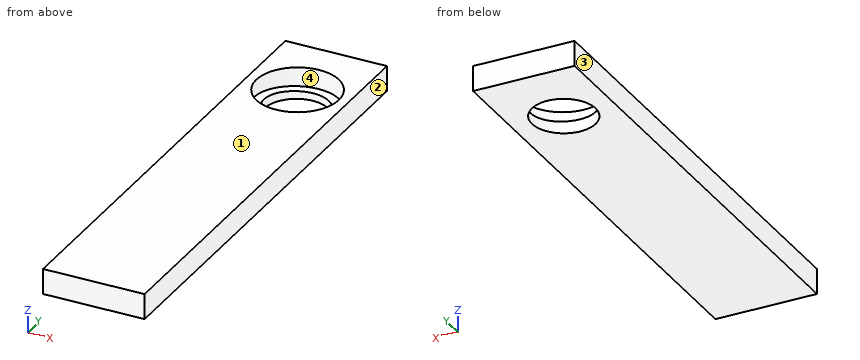
from build123d import *

# Parameters (mm, degrees)
SKETCH1_W           = 80
SKETCH1_H           = 372
BOSS_EXTRUDE1_DEPTH = 20
SKETCH4_R           = 32.5
CUT_EXTRUDE2_DEPTH  = 193.049397179
SKETCH5_R           = 25
CUT_EXTRUDE3_DEPTH  = 193.049397179


with BuildPart() as part:
    # Sketch1 → Boss-Extrude1 (new body)
    with BuildSketch(Plane.XY):
        Rectangle(SKETCH1_W, SKETCH1_H)
    extrude(amount=BOSS_EXTRUDE1_DEPTH)

    # Sketch4 → Cut-Extrude2 (cut, through all)
    with BuildSketch(Plane(origin=(0, 1.135010798, 16.231410618), x_dir=(1, 0, 0), z_dir=(0, -0.06975647374412888, -0.997564050259824))):
        with Locations(Location((0, -124.995505595, 0), (0, 0, 270))):
            Circle(SKETCH4_R)
    extrude(amount=-CUT_EXTRUDE2_DEPTH, mode=Mode.SUBTRACT)

    # Sketch5 → Cut-Extrude3 (cut, through all)
    with BuildSketch(Plane(origin=(0, 1.135010798, 16.231410618), x_dir=(1, 0, 0), z_dir=(0, 0.06975647374412888, 0.9975640502598241))):
        with Locations(Location((0, 124.297940858, 0), (0, 0, 270))):
            Circle(SKETCH5_R)
    extrude(amount=-CUT_EXTRUDE3_DEPTH, mode=Mode.SUBTRACT)


solid = part.part
The model under review builds one solid part; all positions refer to its coordinate system, in mm. Face numbers are marked on the shaded views. Round coordinates to 2 decimals unless told otherwise and drop trailing zeros. Write each loop counter-clockwise with the first axis right and the second up, starting at its lowest first coordinate (ties: lowest second). Pieces come first, ordered by that corner, then holes. Notation, with made-up numbers: (44, -30.5) - (68, -30.5) arc R11 ccw to (68, -12.5) - close; hole circle Ø11 at (35.25, 57.5). An arc over 180 degrees is marked (long way). One line per item, written item: value. Start each with the question number.
1. Consider section B-B on x = -17.5. Write out the cut boundary in (y, z), and give its area (3 significant figures).
2. To check wall thickness, follow L1, parallel to Y at x = 20, z = 11.75; L2, parallel to Y at x = 6, z = 2.5; L3, parallel to X at y = 98, z = 11.75. State the ranges of each line that lie inside material, in increasing order. Write a range as from..to.
3. Consider section A-A on x = 18. Write out the cut boundary in (y, z), and give its area (3 significant figures).
4. The part is to be moulded in two halves that separate along X. For the marked faces 1, 2, 3 and 4, say which applies: released by +X, released by -X, zero draft, split by the parting line, or undercut.
Checks:
1. outline: (-186, 0) - (106.7, 0) - (107.32, 8.81) - (98.51, 9.42) - (99.25, 20) - (-186, 20) - close; (142.5, 0) - (186, 0) - (186, 20) - (154.15, 20) - (153.15, 5.6) - (142.94, 6.32) - close
1. area: 6,480 mm^2
2. L1: y = -186..100.44, 151.8..186
2. L2: y = -186..100.45, 149.1..186
2. L3: x = -40..-16.41, 16.41..40
3. outline: (-186, 0) - (107.21, 0) - (107.82, 8.77) - (98.83, 9.4) - (99.57, 20) - (-186, 20) - close; (141.99, 0) - (186, 0) - (186, 20) - (153.83, 20) - (152.82, 5.62) - (142.44, 6.35) - close
3. area: 6,500 mm^2
4. face 1: zero draft
4. face 2: released by +X
4. face 3: released by -X
4. face 4: undercut
